CAD build for the part. Positions are in the model's coordinates, mm. Face numbers are marked on the shaded views. A direction names the side the tool comes from. Coordinates: 2 decimals unless noted, no trailing zeros. Order: outer loops, then holes, each group sorted by start corner. A loop starts at its lowest first (then second) coordinate and runs counter-clockwise, first axis right, second up. Notation, with made-up numbers: (1.5, 18) - (60.5, 18) arc R23 ccw to (60.5, 54) - close; hole circle Ø8 at (9.25, 2.25). An arc over 180 degrees is marked (long way). Write each question's results on one line, items separated by ' | '. Start each with the question number.
Q1. Which spindle directions (+Z, -Z, +X, -X, +Y, -Y) get a long thin tool onto all of the face, cutting with end or side? Do the marked faces 1, 2 and 3. Say none if no direction does.
Q2. Band-saw the part on B-B, the plane z = 12. Write the cut outline in (x, y), then the cut area to 3 significant figures.
Q3. Wall check: probe 1 along Y at (x, z) = (2.5, 8); probe 2 along X at (y, z) = (12.25, 2); probe 3 along Y at (x, z) = (-1, 0.5). Give the ranges that are in metal, low to high.
Q4. Pin check, flat tips, straight feed: P1, Ø1.4, axis at x = -13, y = 1, coming from the +Z side; P2, Ø2, axis at y = 1.5, z = 11.5, coming from the +X side; P3, Ø10, axis at x = 0, y = 13.5, coming from the +Z side; P4, Ø4, axis at x = -7.5, y = 13.5, coming from the +Z side. Stop position of each tip, or through.
Q5. Band-saw the part on A-A, the plane x = -14.5. Write the cut outline in (y, z).
Q6. Pull direction Z, two halves, no side cores. Call the marked faces 4, 5 and 6: released by +Z, released by -Z, zero draft, split by the parting line, or undercut.
Q7. Band-saw the part on C-C, the plane y = 7.5. Write the cut outline in (x, z).
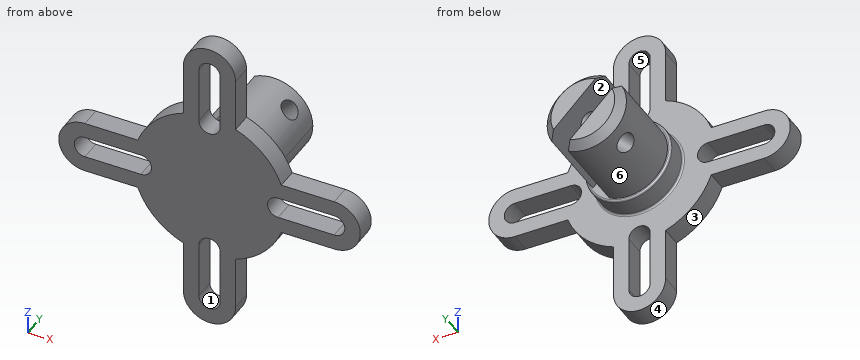
```python
from build123d import *

# Parameters (mm, degrees)
SKETCH3_R                      = 10.033
BOSS_EXTRUDE1_DEPTH            = 2.7432
BOSS_EXTRUDE2_START            = -2.7432
BOSS_EXTRUDE2_DEPTH            = 2.7432
CUT_EXTRUDE1_REACH             = 24.376
CIRPATTERN1_COUNT              = 4
SKETCH5_R                      = 5.6515
BOSS_EXTRUDE3_DEPTH            = 2.921
BOSS_EXTRUDE4_DEPTH            = 11.303
CHAMFER1_SIZE                  = 1.016
FILLET1_R                      = 0.254
CUT_EXTRUDE2_REACH             = 36.085
SKETCH7_R                      = 1.27
CUT_EXTRUDE2_DIRECTION_2_REACH = 36.085


with BuildPart() as part:
    # Sketch3 → Boss-Extrude1 (new body)
    with BuildSketch(Plane(origin=(0, 0, 0), x_dir=(1, 0, 0), z_dir=(0, 1, 0))):
        with Locations(Location((0, 0, 0), (0, 0, 270))):
            Circle(SKETCH3_R)
    extrude(amount=BOSS_EXTRUDE1_DEPTH)

    # Sketch4 → Boss-Extrude2 (add)
    with BuildSketch(Plane(origin=(0, 2.7432, 0), x_dir=(1, 0, 0), z_dir=(0, 1, 0)).offset(BOSS_EXTRUDE2_START)):
        with BuildLine():
            ThreePointArc((9.428841286, 3.429), (9.73521463, 2.426249185), (9.935264466, 1.397))
            Line((9.935264466, 1.397), (16.383, 1.397))
            ThreePointArc((16.383, 1.397), (17.78, 0), (16.383, -1.397))
            Line((16.383, -1.397), (9.935264466, -1.397))
            ThreePointArc((9.935264466, -1.397), (9.73521463, -2.426249185), (9.428841286, -3.429))
            Line((9.428841286, -3.429), (16.383, -3.429))
            ThreePointArc((16.383, -3.429), (19.812, 0), (16.383, 3.429))
            Line((16.383, 3.429), (9.428841286, 3.429))
        make_face()
    boss_extrude2 = extrude(amount=BOSS_EXTRUDE2_DEPTH)

    # Sketch4<3> → Cut-Extrude1 (cut, up to next)
    with BuildSketch(Plane(origin=(0, 2.7432, 0), x_dir=(1, 0, 0), z_dir=(0, 1, 0)), mode=Mode.PRIVATE) as cut_extrude1_sk1:
        with BuildLine():
            Line((9.935264466, 1.397), (9.017, 1.397))
            ThreePointArc((9.017, 1.397), (7.62, 0), (9.017, -1.397))
            Line((9.017, -1.397), (9.935264466, -1.397))
            ThreePointArc((9.935264466, -1.397), (10.008536291, -0.700207333), (10.033, 0))
            ThreePointArc((10.033, 0), (10.008536291, 0.700207333), (9.935264466, 1.397))
        make_face()
    cut_extrude1_tool1 = extrude(cut_extrude1_sk1.sketch, amount=-CUT_EXTRUDE1_REACH, mode=Mode.PRIVATE) & part.part
    cut_extrude1 = cut_extrude1_tool1.solids().sort_by_distance((8.936983, 2.7432, 0))[0]
    add(cut_extrude1, mode=Mode.SUBTRACT)

    # CirPattern1: Boss-Extrude2, Cut-Extrude1 ×4 about axis
    cirpattern1_axis = Axis((0, 0, 0), (0, 1, 0))
    add([boss_extrude2.rotate(cirpattern1_axis, i * 360 / CIRPATTERN1_COUNT) for i in range(1, CIRPATTERN1_COUNT)])
    add([cut_extrude1.rotate(cirpattern1_axis, i * 360 / CIRPATTERN1_COUNT) for i in range(1, CIRPATTERN1_COUNT)], mode=Mode.SUBTRACT)

    # Sketch5 → Boss-Extrude3 (add)
    with BuildSketch(Plane(origin=(0, 2.7432, 0), x_dir=(1, 0, 0), z_dir=(0, 1, 0))):
        with Locations(Location((0, 0, 0), (0, 0, 270))):
            Circle(SKETCH5_R)
    extrude(amount=BOSS_EXTRUDE3_DEPTH)

    # Sketch6 → Boss-Extrude4 (add)
    with BuildSketch(Plane(origin=(0, 5.6642, 0), x_dir=(1, 0, 0), z_dir=(0, 1, 0))):
        with BuildLine():
            ThreePointArc((5.207, 0), (5.054935189, 1.249191434), (4.607622532, 2.425420294))
            Line((4.607622532, 2.425420294), (-2.425420294, -4.607622532))
            ThreePointArc((-2.425420294, -4.607622532), (2.691067216, -4.457690684), (5.207, 0))
        make_face()
        with BuildLine():
            Line((-4.607622532, -2.425420294), (2.425420294, 4.607622532))
            ThreePointArc((2.425420294, 4.607622532), (-3.68190501, 3.68190501), (-4.607622532, -2.425420294))
        make_face()
    extrude(amount=BOSS_EXTRUDE4_DEPTH)

    # Chamfer1
    chamfer1_edges = [part.edges().sort_by_distance(p)[0] for p in [
        (3.68190501, 16.9672, 3.68190501),
        (-3.68190501, 16.9672, -3.68190501),
    ]]
    chamfer(chamfer1_edges, length=CHAMFER1_SIZE)

    # Fillet1
    fillet1_edges = [part.edges().sort_by_distance(p)[0] for p in [
        (0, 2.7432, -5.6515),
        (0, 5.6642, -5.6515),
    ]]
    fillet(fillet1_edges, radius=FILLET1_R)

    # Sketch7 → Cut-Extrude2 (cut, up to next)
    with BuildSketch(Plane(origin=(-1.091101119, 0, -1.091101119), x_dir=(0.7071067811865486, 0, -0.7071067811865465), z_dir=(0.7071067811865465, 0, 0.7071067811865486)), mode=Mode.PRIVATE) as cut_extrude2_sk1:
        with Locations(Location((0, 13.1572, 0), (0, 0, 180))):
            Circle(SKETCH7_R)
    cut_extrude2_tool1 = extrude(cut_extrude2_sk1.sketch, amount=-CUT_EXTRUDE2_REACH, mode=Mode.PRIVATE) & part.part
    add(cut_extrude2_tool1.solids().sort_by_distance((-1.091101, 13.1572, -1.091101))[0], mode=Mode.SUBTRACT)

    # Sketch7 → Cut-Extrude2 direction 2 (cut, up to next)
    with BuildSketch(Plane(origin=(-1.091101119, 0, -1.091101119), x_dir=(0.7071067811865486, 0, -0.7071067811865465), z_dir=(0.7071067811865465, 0, 0.7071067811865486)), mode=Mode.PRIVATE) as cut_extrude2_direction_2_sk1:
        with Locations(Location((0, 13.1572, 0), (0, 0, 180))):
            Circle(SKETCH7_R)
    cut_extrude2_direction_2_tool1 = extrude(cut_extrude2_direction_2_sk1.sketch, amount=CUT_EXTRUDE2_DIRECTION_2_REACH, mode=Mode.PRIVATE) & part.part
    add(cut_extrude2_direction_2_tool1.solids().sort_by_distance((-1.091101, 13.1572, -1.091101))[0], mode=Mode.SUBTRACT)


solid = part.part
```
Results below:
1) face 1: +Y, -Y | face 2: +Y | face 3: -Z, -X, +Y, -Y
2) outline: (-3.43, 0) - (-1.4, 0) - (-1.4, 2.74) - (-3.43, 2.74) - close; (1.4, 0) - (3.43, 0) - (3.43, 2.74) - (1.4, 2.74) - close | area: 11.1 mm²
3) probe 1: y = 0 to 2.74 | probe 2: x = -4.81 to -4.18, 0.18 to 0.74, 3.26 to 4.81 | probe 3: y = 0 to 5.66
4) P1: stops at z = 3.43 | P2: stops at x = 3.43 | P3: stops at z = 5.21 | P4: passes through
5) outline: (0, -3.43) - (2.74, -3.43) - (2.74, -1.4) - (0, -1.4) - close; (0, 1.4) - (2.74, 1.4) - (2.74, 3.43) - (0, 3.43) - close
6) face 4: released by -Z | face 5: undercut | face 6: split by the parting line
7) outline: (-4.61, 2.43) arc R5.21 ccw to (2.43, -4.61) - close; (-2.43, 4.61) - (4.61, -2.43) arc R5.21 ccw to start
